```python
from build123d import *

# Parameters (mm, degrees)
HOLE_WIZARD_M22_D           = 2
HOLE_WIZARD_M22_CSINK_D     = 4.4
HOLE_WIZARD_M22_CSINK_ANGLE = 90
PATTERN_CIRCULAR_2_COUNT    = 4
SKETCH_6_R                  = 3.5
EXTRUDE_1_DEPTH             = 17
SKETCH_7_R                  = 14
EXTRUDE_2_DEPTH             = 3
CUT_EXTRUDE_1_REACH         = 35.481
SKETCH_8_R                  = 1
PATTERN_CIRCULAR_3_COUNT    = 4


with BuildPart() as part:
    # Sketch 1 → Revolve 1 (revolve)
    with BuildSketch(Plane.XY, mode=Mode.PRIVATE) as revolve_1_sk:
        Polygon((0, 10), (0, 11), (7, 11), (7, 0), (4, 0), (4, 10), align=None)
    revolve(revolve_1_sk.sketch.rotate(Axis((0, 0, 0), (1, 0, 0)), 90), axis=Axis((0, 0, 0), (1, 0, 0)))

    # Hole Wizard M22 (through all)
    with Locations(Plane(origin=(7, 0, 0), x_dir=(0, 0, -1), z_dir=(1, 0, 0))):
        with Locations((-2.933383142, 5.234048466)):
            hole_wizard_m22 = CounterSinkHole(HOLE_WIZARD_M22_D / 2, HOLE_WIZARD_M22_CSINK_D / 2, counter_sink_angle=HOLE_WIZARD_M22_CSINK_ANGLE)

    # Pattern Circular 2: Hole Wizard M22 ×4 about axis
    pattern_circular_2_axis = Axis((0, 0, 0), (1, 0, 0))
    for i in range(1, PATTERN_CIRCULAR_2_COUNT):
        add(hole_wizard_m22.rotate(pattern_circular_2_axis, i * 360 / PATTERN_CIRCULAR_2_COUNT), mode=Mode.SUBTRACT)

    # Sketch 6 → Extrude 1 (add)
    with BuildSketch(Plane(origin=(7, 0, 0), x_dir=(0, 0, -1), z_dir=(1, 0, 0))):
        with Locations(Location((0, 0, 0), (0, 0, 180))):
            Circle(SKETCH_6_R)
    extrude(amount=EXTRUDE_1_DEPTH)

    # Sketch 7 → Extrude 2 (add)
    with BuildSketch(Plane(origin=(24, 0, 0), x_dir=(0, 0, -1), z_dir=(1, 0, 0))):
        Circle(SKETCH_7_R)
    extrude(amount=EXTRUDE_2_DEPTH)

    # Sketch 8 → Cut-Extrude 1 (cut, up to next)
    with BuildSketch(Plane(origin=(27, 0, 0), x_dir=(0, 0, -1), z_dir=(1, 0, 0)), mode=Mode.PRIVATE) as cut_extrude_1_sk1:
        with Locations((-5.499090834, 7.5)):
            Circle(SKETCH_8_R)
    cut_extrude_1_tool1 = extrude(cut_extrude_1_sk1.sketch, amount=-CUT_EXTRUDE_1_REACH, mode=Mode.PRIVATE) & part.part
    cut_extrude_1 = cut_extrude_1_tool1.solids().sort_by_distance((27, 7.5, 5.499091))[0]
    add(cut_extrude_1, mode=Mode.SUBTRACT)

    # Pattern Circular 3: Cut-Extrude 1 ×4 about axis
    pattern_circular_3_axis = Axis((0, 0, 0), (1, 0, 0))
    for i in range(1, PATTERN_CIRCULAR_3_COUNT):
        add(cut_extrude_1.rotate(pattern_circular_3_axis, i * 360 / PATTERN_CIRCULAR_3_COUNT), mode=Mode.SUBTRACT)


solid = part.part
```
Design review of the part built by this model. Coordinates are the model's own, in mm. A direction names the side the tool comes from. Coordinates: 2 decimals unless noted, no trailing zeros. Write each loop counter-clockwise with the first axis right and the second up, starting at its lowest first coordinate (ties: lowest second). Pieces come first, ordered by that corner, then holes.
1) Mouldability with a two-part tool opening along Y and no side actions: class faces 1 (the flat face through (7, -2.6, -2.6)), 2 (the cylindrical face through (25.521, -4.545, 7.8)), 3 (the cylindrical face through (4.887, -3.395, 4.347)), 4 (the cylindrical face through (3.55, 10.74, -2.38)) as +Y half, -Y half, draft (parallel to the pull), parting line (faces both ways), or undercut.
2) Machinability: for faces 5 (the flat face through (24, -3, -3)), 6 (the cylindrical face through (2, 0, -10)), 7 (the cylindrical face through (25.521, 4.545, -7.8)), which of the approach directions +Z, -Z, +X, -X, +Y, -Y give a long, thin tool a straight path to every point of the face, cutting with its end or side? Answer none if there is none.
3) Insertion check: pin 1 (4 mm diameter, centred on x = 14.5, y = -1, fed in from +Z); pin 2 (3 mm diameter, centred on y = -4, z = -2.5, fed in from -X); pin 3 (4 mm diameter, centred on x = 4.5, y = -8, fed in from +Z). Each pin has a flat end and moves straight along its axis. Give the tip position at first contact, or say it passes through.
4) Add section B-B (y = 0). Write out the cut boundary in (x, z).
5) Add section A-A (y = -10.5). Write out the cut boundary in (x, z).
6) To check wall thickness, follow L1, parallel to X at y = 7.75, z = 0; L2, parallel to Y at x = 3, z = 0; L3, parallel to X at y = 9.5, z = -3.5. State the ranges of each line that lie inside material, in increasing order.
Check result:
1. face 1: draft
1. face 2: undercut
1. face 3: undercut
1. face 4: parting line
2. face 5: none
2. face 6: -X
2. face 7: +X
3. pin 1: stops at z = 3.5
3. pin 2: stops at x = 4
3. pin 3: stops at z = 9.22
4. outline: (0, -11) - (7, -11) - (7, -3.5) - (24, -3.5) - (24, -14) - (27, -14) - (27, 14) - (24, 14) - (24, 3.5) - (7, 3.5) - (7, 11) - (0, 11) - (0, 10) - (4, 10) - (4, -10) - (0, -10) - close
5. outline: (0, -3.28) - (7, -3.28) - (7, 3.28) - (0, 3.28) - close; (24, -9.26) - (27, -9.26) - (27, 9.26) - (24, 9.26) - close
6. L1: x = 4 to 7, 24 to 27
6. L2: y = -11 to -10, 10 to 11
6. L3: x = 0 to 7, 24 to 27
